Geometry: final body of the model. Coordinates: model frame, mm. A direction names the side the tool comes from. Give positions to 0.01 mm unless a question says otherwise; leave off trailing zeros. Order: outer loops, then holes, each group sorted by start corner. A loop starts at its lowest first (then second) coordinate and runs counter-clockwise, first axis right, second up. Notation, with made-up numbers: M 65,3 L 101,3 A25 cw 101,38 Z; hole C -33.75,38 d1. An arc over 180 degrees is marked long. One line per item, written item: value. Start each with the question number.
```python
from build123d import *

# Parameters (mm, degrees)
F0_R     = 6.95
F1_DEPTH = 25
F2_W     = 46
F2_H     = 76.95
F2_R     = 6.95
F3_DEPTH = 40
F5_DEPTH = 76.951
F6_R     = 6
F7_DEPTH = 46.001


with BuildPart() as f1:
    # F0 (on Right) → F1 (new body)
    with BuildSketch(Plane.YZ):
        Circle(F0_R)
    extrude(amount=-F1_DEPTH)

    # F2 (on Right) → F3 (join)
    with BuildSketch(Plane.YZ):
        with Locations((0, 26.525)):
            Rectangle(F2_W, F2_H)
        Circle(F2_R, mode=Mode.SUBTRACT)
        Circle(F2_R)
    extrude(amount=F3_DEPTH)

    # F4 (on face) → F5 (cut, through all)
    with BuildSketch(Plane.XY.offset(65)):
        with BuildLine():
            Line((40, -18), (40, 18))
            Line((40, 18), (15, 18))
            ThreePointArc((15, 18), (7.928932, 15.071068), (5, 8))
            Line((5, 8), (5, -8))
            ThreePointArc((5, -8), (7.928932, -15.071068), (15, -18))
            Line((15, -18), (40, -18))
        make_face()
    extrude(amount=-F5_DEPTH, mode=Mode.SUBTRACT)

    # F6 (on face) → F7 (cut, through all)
    with BuildSketch(Plane.XZ.offset(23)):
        with BuildLine():
            Line((40, 50), (40, 65))
            Line((40, 65), (25, 65))
            ThreePointArc((25, 65), (35.606602, 60.606602), (40, 50))
        make_face()
        with BuildLine():
            Line((40, -11.95), (40, 47.164207))
            Line((40, 47.164207), (38.964771, 44.524128))
            Line((38.964771, 44.524128), (19.309847, -5.600581))
            ThreePointArc((19.309847, -5.600581), (15.634456, -10.211532), (10, -11.95))
            Line((10, -11.95), (40, -11.95))
        make_face()
        with Locations((25, 50)):
            Circle(F6_R)
    extrude(amount=-F7_DEPTH, mode=Mode.SUBTRACT)


solid = f1.part
```
Q1. Mould query, pull axis X, two halves, no side actions, for faces 4 (the face through (-25, 0, 0)), 5 (the face through (20.24, -20.54, 46.35)), 6 (the face through (15, 23, 26)), 7 (the face through (15.703, 20.49, -10.164)). Classes: +X half, -X half, draft (parallel to the pull), parting line (faces both ways), or undercut.
Q2. Section query C-C on x = 8. Return loops of the section in (y, z), and give its area (3 significant figures).
Q3. Section query B-B on z = 48.5. Return loops of the section in (x, y), and give its area (3 significant figures).
Q4. Section query D-D on z = -3. Return loops of the section in (x, y).
Q5. Contact query for flat-ended pins moving along their axis: pin 1 (12 mm diameter, centred on y = -3.5, z = -1, fed in from +X); pin 2 (8 mm diameter, centred on y = -11, z = 24.5, fed in from +X); pin 3 (6 mm diameter, centred on y = 2.5, z = 24.5, fed in from -X). Output: stop coordinate, or through.
Q6. Section query A-A on y = 0. Return loops of the section in (x, z), and give its area (3 significant figures).
Q7. Set-up query: faces 1 (the face through (-12.325, -1.507, -6.785)), 2 (the face through (35.49, 20.47, 60.72)), 3 (the face through (5, 0, 27)). Return all of +Z, -Z, +X, -X, +Y, -Y with unobstructed straight access to the full face (end or side cutting, diameter ignored); none if empty.
Q8. Ray query, line 1 along Y through (x, z) = (14.5, 23.5); line 2 along Z through (x, y) = (10.5, 19.5); line 3 along X through (y, z) = (3.5, 36). Return the intervals inside material, ascending. Write a range as [from, to].
Results below:
1. face 4: -X half
1. face 5: undercut
1. face 6: draft
1. face 7: +X half
2. outline: M -23,-11.95 L -15.14,-11.95 L -15.14,65 L -23,65 Z; M 15.14,-11.95 L 23,-11.95 L 23,65 L 15.14,65 Z
2. area: 1,210 mm2
3. outline: M 0,-23 L 19.19,-23 L 19.19,-18 L 15,-18 A10 cw 5,-8 L 5,8 A10 cw 15,18 L 19.19,18 L 19.19,23 L 0,23 Z; M 30.81,-23 L 40,-23 L 40,-18 L 30.81,-18 Z; M 30.81,18 L 40,18 L 40,23 L 30.81,23 Z
3. area: 507 mm2
4. outline: M -25,-6.27 L 0,-6.27 L 0,-23 L 20.33,-23 L 20.33,-18 L 15,-18 A10 cw 5,-8 L 5,8 A10 cw 15,18 L 20.33,18 L 20.33,23 L 0,23 L 0,6.27 L -25,6.27 Z
5. pin 1: x = 5.11
5. pin 2: x = 7.86
5. pin 3: x = 0
6. outline: M -25,-6.95 L 0,-6.95 L 0,-11.95 L 5,-11.95 L 5,65 L 0,65 L 0,6.95 L -25,6.95 Z
6. area: 732 mm2
7. face 1: -X
7. face 2: +Z, +X, +Y, -Y
7. face 3: +Z, -Z, +X
8. line 1: [-23, -17.99], [17.99, 23]
8. line 2: [-11.94, 65]
8. line 3: [0, 5]
